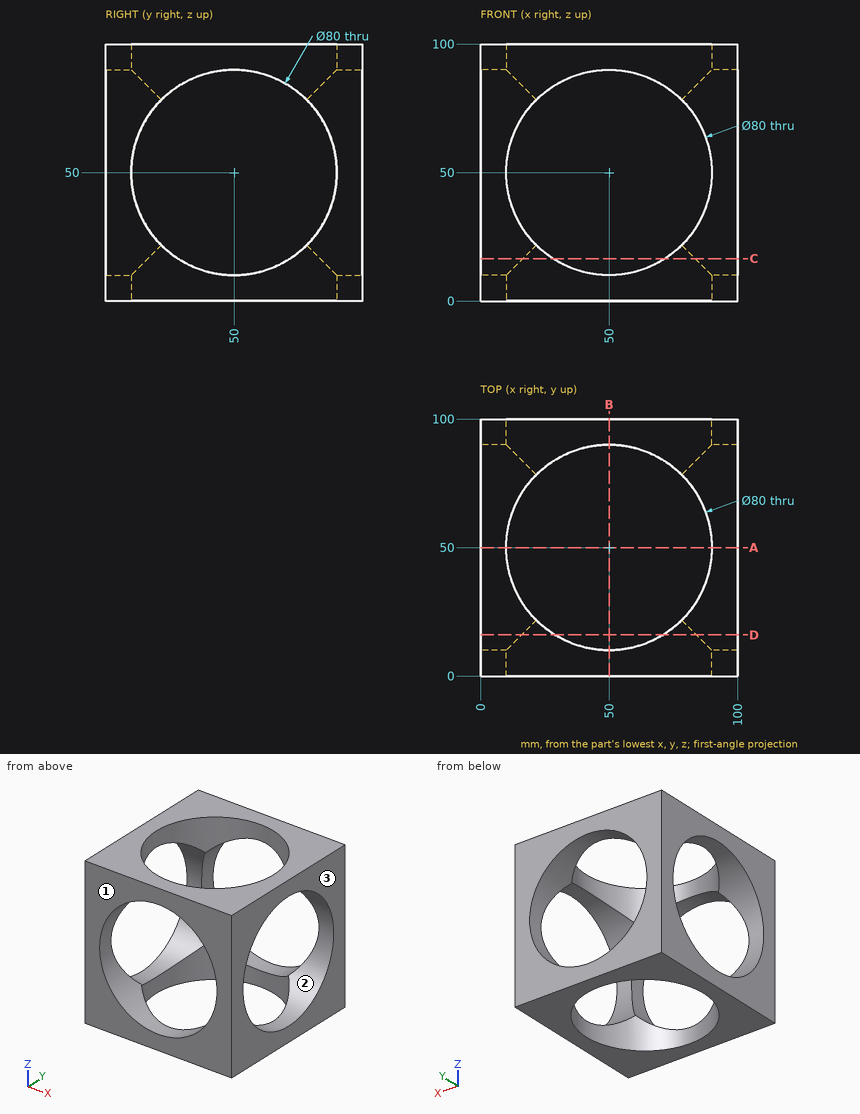
Study the drawing (mm; zero at the part's minimum x, y, z) and answer. Give positions to 0.01 mm unless a question says otherwise; leave off trailing zeros. Write each loop counter-clockwise with the first axis right and the second up, starting at its lowest first coordinate (ties: lowest second). Pieces come first, ordered by that corner, then holes. Notation, with made-up numbers: (0.25, -30) - (58.25, -30) arc R24 cw to (58.25, 6) - close; hole circle Ø6 at (88, 44). An arc over 180 degrees is marked (long way). Write item = value, one per line. Start each with the question number.
Item 1: Find section C-C (z = 16.5). Give the vertices of the cut face in (x, y), then the cut area to 3 significant figures.
Item 2: The mould has two halves that part along Y. Classify the marked faces 1, 2 and 3: +Y half, -Y half, draft (parallel to the pull), parting line (faces both ways), or undercut.
Item 3: Find section A-A (y = 50). Give the vertices of the cut face in (x, z).
Item 4: Find section D-D (y = 16). Give the vertices of the cut face in (x, z), then the cut area to 3 significant figures.
Item 5: Find the intervals of material crossed by probe 1 along Z at (x, y) = (12, 72); probe 2 along Z at (x, y) = (95, 50); probe 3 along X at (y, z) = (37, 10), in increasing order. Write a range as [from, to].
Response:
q1.outline = (0, 0) - (28.14, 0) - (28.14, 16.5) arc R40 cw to (16.5, 28.14) - (0, 28.14) - close; (0, 71.86) - (16.5, 71.86) arc R40 cw to (28.14, 83.5) - (28.14, 100) - (0, 100) - close; (71.86, 0) - (100, 0) - (100, 28.14) - (83.5, 28.14) arc R40 cw to (71.86, 16.5) - close; (71.86, 83.5) arc R40 cw to (83.5, 71.86) - (100, 71.86) - (100, 100) - (71.86, 100) - close
q1.area = 2,860 mm²
q2.face_1 = -Y half
q2.face_2 = undercut
q2.face_3 = draft
q3.outline = (0, 0) - (10, 0) - (10, 10) - (0, 10) - close; (0, 90) - (10, 90) - (10, 100) - (0, 100) - close; (90, 0) - (100, 0) - (100, 10) - (90, 10) - close; (90, 90) - (100, 90) - (100, 100) - (90, 100) - close
q4.outline = (0, 0) - (28.93, 0) - (28.93, 16) arc R40 cw to (16, 28.93) - (0, 28.93) - close; (0, 71.07) - (16, 71.07) arc R40 cw to (28.93, 84) - (28.93, 100) - (0, 100) - close; (71.07, 0) - (100, 0) - (100, 28.93) - (84, 28.93) arc R40 cw to (71.07, 16) - close; (71.07, 84) arc R40 cw to (84, 71.07) - (100, 71.07) - (100, 100) - (71.07, 100) - close
q4.area = 2,960 mm²
q5.probe_1 = [0, 16.59], [83.41, 100]
q5.probe_2 = [0, 10], [90, 100]
q5.probe_3 = [0, 12.17], [87.83, 100]
